Read the model definition and answer for the solid it produces. Units are mm, in the model's axes. Face numbers are marked on the shaded views. A direction names the side the tool comes from. Give positions to 0.01 mm unless a question says otherwise; leave off trailing zeros. Order: outer loops, then holes, each group sorted by start corner. A loop starts at its lowest first (then second) coordinate and runs counter-clockwise, first axis right, second up. Notation, with made-up numbers: (-11, 64.5) -> (46, 64.5) arc R19 cw to (46, 97.5) -> close; hole circle Ø4 at (76, -17). An arc over 180 degrees is marked (long way). Use one line per item in the form item = value.
Solid Edge part; units mm, degrees
sketch "Sketch1" plane through (0, 0, 0) normal (0, -1, 0) x (1, 0, 0)
  line L0 (2.5, 0) -> (5, 2.5)
  line L1 (5, 2.5) -> (5, 2.8)
  line L2 (5, 2.8) -> (0, 2.8)
  line L3 (0, 2.8) -> (0, -57.2)
  line L4 (0, -57.2) -> (2.0095, -57.2)
  line L5 (2.0095, -57.2) -> (2.5, -56.7095)
  line L6 (2.5, -56.7095) -> (2.5, -41.2)
  line L7 (2.5, -41.2) -> (2.0095, -41.2)
  line L8 (2.0095, -41.2) -> (2.0095, -41.19)
  line L9 (2.0095, -41.19) -> (2.5, -41.19)
  line L10 (2.5, -41.19) -> (2.5, 0)
  dimension "D1" = 2.5
  dimension "D2" = 2.0095
revolve "RevolvedProtrusion1" add sketch "Sketch1" angle 360 about axis through (0, 0, 54) along (0, 0, -1)
sketch "Sketch2" plane through (0, 0, 0) normal (0, -1, 0) x (1, 0, 0)
  arc A0 (-1.5, 0.5) -> (0, 0) centre (0, 2.5) ccw
  line L0 (0, 0.5) -> (0, 0)
  line L1 (-1.5, 0.5) -> (0, 0.5)
revolve "RevolvedCutout1" cut sketch "Sketch2" angle 360 about axis through (0, 0, 54) along (0, 0, -1)
sketch "Sketch3" plane through (0, 0, 2.8) normal (0, 0, 1) x (0, -1, 0)
  line L0 (-1.7321, 0) -> (-0.866, 1.5)
  line L1 (-0.866, 1.5) -> (0.866, 1.5)
  line L2 (0.866, 1.5) -> (1.7321, 0)
  line L3 (1.7321, 0) -> (0.866, -1.5)
  line L4 (0.866, -1.5) -> (-0.866, -1.5)
  line L5 (-0.866, -1.5) -> (-1.7321, 0)
extrude "Cutout1" cut sketch "Sketch3" against normal blind 2.3
cosmetic_thread "Thread1"
sketch "Sketch4" plane through (0, 0, 0) normal (1, 0, 0) x (0, 1, 0)
  line L0 (-1.72, 2.8) -> (0, 1.807)
revolve "RevolvedCutout2" cut sketch "Sketch4" angle 360 about axis through (0, 0, -57) along (0, 0, 1) material side at (0, -0.835, 2.3468)
fillet "Round1" radius 0.2 1 edges at (-2.5, 0, 0)
properties material "Stahl"
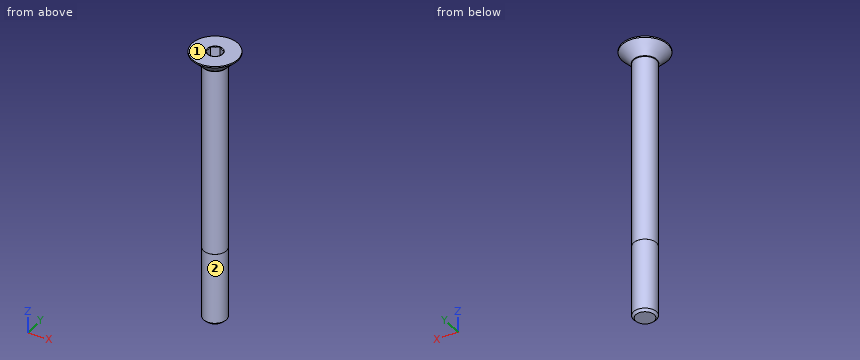
Item 1: Given pin 1 Ø3 at (x, z) = (-3, -35) entering from +Y; pin 2 Ø0.5 at (x, y) = (0.5, -1) entering from +Z; pin 3 Ø1.5 at (y, z) = (0.5, -13.5) entering from -X, each flat-ended and moving along its own axis, determine where each tip first touches the part or whether it passes through.
Checks:
pin_1 = 2
pin_2 = 0.41
pin_3 = -2.5
Item 2: Which of the six approach directions +Z, -Z, +X, -X, +Y, -Y give full straight-line access (tool end or side, diameter ignored) to the marked faces 1 and 2?
Checks:
face_1 = +Z, +X, -X, +Y, -Y
face_2 = -Z
Item 3: The part is cut by section A-A on z = -35. Give the vertices of the cut face in (x, y), and give its area (3 significant figures).
Checks:
outline = circle Ø5 at (0, 0)
area = 19.6 mm²
Item 4: Straight lines are drawn through the part: L1, parallel to X at y = 0, z = -17; L2, parallel to Y at x = 1.5, z = -41; L3, parallel to X at y = 2, z = -29. For each, find the intervals that lie inside material, in ascending order. Write a range as from..to.
Checks:
L1 = -2.5..2.5
L2 = -2..2
L3 = -1.5..1.5
